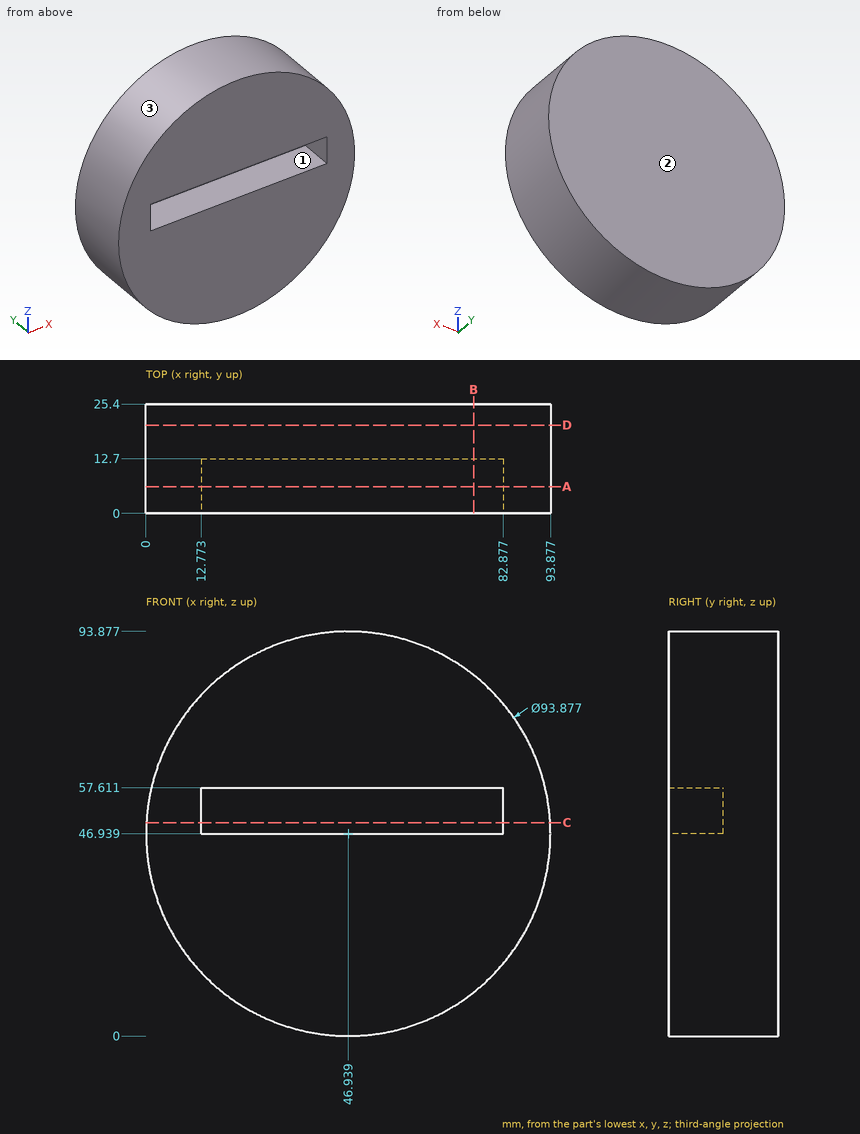
Print and shaded views of the part. All mm, measured from the part's lowest x, y and z. Coordinates: 2 decimals unless noted, no trailing zeros. Order: outer loops, then holes, each group sorted by start corner. A loop starts at its lowest first (then second) coordinate and runs counter-clockwise, first axis right, second up. Notation, with made-up numbers: (-7, -2) -> (40, -2) arc R15 cw to (40, 15) -> close; hole circle Ø1 at (41, 29). An arc over 180 degrees is marked (long way). Answer as a JSON object with one key per item and string values. Group by question number.
1) Pull direction Z, two halves, no side cores. Call the marked faces 1, 2 and 3: +Z half, -Z half, draft (parallel to the pull), parting line (faces both ways), or undercut.
2) Cut at A-A, the plane y = 6.25. Write the cut outline in (x, z).
3) Cut at C-C, the plane z = 49.5. Write the cut outline in (x, y), then the cut area to 3 significant figures.
4) Cut at B-B, the plane x = 76. Write the cut outline in (y, z).
5) Flat gauge pins, fed straight in: pin 1 (5.5 mm diameter, centred on x = 49, z = 52, fed in from -Y); pin 2 (3 mm diameter, centred on x = 59, y = 8.5, fed in from -Z); pin 3 (6 mm diameter, centred on y = 7.5, z = 67.5, fed in from -X). Where does each tip first touch, or does it go through?
6) Drill centre lines: L1, parallel to Z at x = 21, y = 4.75; L2, parallel to Z at x = 67, y = 4.5 (1 decimal); L3, parallel to X at y = 4.5, z = 41.5. Where is each one in solid material? Low to high.
7) Cut at D-D, the plane y = 20.5. Write the cut outline in (x, z).
Check values:
{
 "1": {"face 1": "undercut", "face 2": "draft", "face 3": "parting line"},
 "2": {"outline": "circle Ø93.88 at (46.94, 46.94); hole (12.77, 46.94) -> (82.88, 46.94) -> (82.88, 57.61) -> (12.77, 57.61) -> close"},
 "3": {"outline": "(0.07, 0) -> (12.77, 0) -> (12.77, 12.7) -> (82.88, 12.7) -> (82.88, 0) -> (93.81, 0) -> (93.81, 25.4) -> (0.07, 25.4) -> close", "area": "1,490 mm²"},
 "4": {"outline": "(0, 10.08) -> (25.4, 10.08) -> (25.4, 83.8) -> (0, 83.8) -> (0, 57.61) -> (12.7, 57.61) -> (12.7, 46.94) -> (0, 46.94) -> close"},
 "5": {"pin 1": "stops at y = 12.7", "pin 2": "stops at z = 1.2", "pin 3": "stops at x = 3.41"},
 "6": {"L1": "z = 7.82 to 46.94, 57.61 to 86.06", "L2": "z = 4.5 to 46.9, 57.6 to 89.4", "L3": "x = 0.32 to 93.56"},
 "7": {"outline": "circle Ø93.88 at (46.94, 46.94)"}
}
